Geometry: final body of the model. Coordinates: model frame, mm. A direction names the side the tool comes from. Round coordinates to 2 decimals unless told otherwise and drop trailing zeros. Loops run counter-clockwise (first coordinate to the right, second up) from the corner with the lowest first, then second, coordinate; pieces in that order, holes last. Notation, with made-up numbers: (16, 74) - (63, 74) arc R21 ccw to (63, 100) - close; hole circle Ø9 at (40.25, 81.25). An arc over 180 degrees is marked (long way). Answer as a JSON object with one key per item and string values. Group by question number.
Item 1: Section D-D (y = -3). Return the cut outline in (x, z).
Item 2: First-contact query: pin 1 (1 mm diameter, centred on x = -45, y = -4, fed in from +Z); pin 2 (1.5 mm diameter, centred on y = 30.5, z = 13, fed in from +X). Flat tips, straight axial feed; report the tip coordinate or a pass-through.
Item 3: Reachability of faces 4 (the face through (3.847, 40.286, 10.14)), 5 (the face through (-15, 38.5, 14)) from +Z, -Z, +X, -X, +Y, -Y: full face, straight path, thin tool, end or side. Return the list, or none.
Item 4: Section B-B (z = 10). Return the cut outline in (x, y).
Item 5: Line query: line 1 (Y direction, x = -22, z = 8.25); line 2 (Z direction, x = 2.5, y = -1); line 3 (X direction, y = 33.5, z = 13.5). Output: solid intervals per line, ascending.
Item 6: Section C-C (x = -7.5). Return the cut outline in (y, z).
Item 7: Section A-A (y = -41.75). Return the cut outline in (x, z).
Item 8: Draft query along X for faces 1 (the face through (-69.828, -1, 10)), 2 (the face through (3.847, -43.214, 10.14)), 3 (the face through (-25, -45, 10)). Return one class per face: released by +X, released by -X, zero draft, split by the parting line, or undercut.
```python
from build123d import *

# Parameters (mm, degrees)
F0_W      = 90
F0_H      = 90
F1_DEPTH  = 20
F2_W      = 70
F2_H      = 77
F3_DEPTH  = 12
F12_R     = 1.5
F13_DEPTH = 25


with BuildPart() as f1:
    # F0 (on Top) → F1 (new body)
    with BuildSketch(Plane.XY):
        with Locations((-24.827586, 0)):
            Rectangle(F0_W, F0_H)
    extrude(amount=F1_DEPTH)

    # F2 (on face) → F3 (cut)
    with BuildSketch(Plane.XY.offset(20)):
        with Locations((-14.827586, 0)):
            Rectangle(F2_W, F2_H)
    extrude(amount=-F3_DEPTH, mode=Mode.SUBTRACT)

    # F4 (on face) → F5 (revolve, cut)
    with BuildSketch(Plane(origin=(0, -38.5, 0), x_dir=(-1, 0, 0), z_dir=(0, 1, 0))):
        with BuildLine():
            Line((32.327586, 11.5), (32.327586, 15.5))
            ThreePointArc((32.327586, 15.5), (30.327586, 13.5), (32.327586, 11.5))
        make_face()
    revolve(axis=Axis((-32.327586, -38.5, 13.5), (0, 0, 1)), mode=Mode.SUBTRACT)

    # F6 (on face) → F7 (revolve, cut)
    with BuildSketch(Plane(origin=(0, -38.5, 0), x_dir=(-1, 0, 0), z_dir=(0, 1, 0))):
        with BuildLine():
            Line((-2.672414, 11.5), (-2.672414, 15.5))
            ThreePointArc((-2.672414, 15.5), (-4.672414, 13.5), (-2.672414, 11.5))
        make_face()
    revolve(axis=Axis((2.672414, -38.5, 13.5), (0, 0, 1)), mode=Mode.SUBTRACT)

    # F8 (on face) → F9 (revolve, cut)
    with BuildSketch(Plane.XZ.offset(-38.5)):
        with BuildLine():
            Line((2.672414, 15.5), (2.672414, 11.5))
            ThreePointArc((2.672414, 11.5), (4.672414, 13.5), (2.672414, 15.5))
        make_face()
    revolve(axis=Axis((2.672414, 38.5, 13.5), (0, 0, 1)), mode=Mode.SUBTRACT)

    # F10 (on face) → F11 (revolve, cut)
    with BuildSketch(Plane.XZ.offset(-38.5)):
        with BuildLine():
            Line((-32.327586, 11.5), (-32.327586, 15.5))
            ThreePointArc((-32.327586, 15.5), (-34.327586, 13.5), (-32.327586, 11.5))
        make_face()
    revolve(axis=Axis((-32.327586, 38.5, 13.5), (0, 0, 1)), mode=Mode.SUBTRACT)

    # F12 (on face) → F13 (cut)
    with BuildSketch(Plane.XY.offset(20)):
        with Locations((4.172414, -41.75)):
            Circle(F12_R)
        with Locations((4.172414, 41.75)):
            Circle(F12_R)
    extrude(amount=-F13_DEPTH, mode=Mode.SUBTRACT)


solid = f1.part
```
Values:
{
 "1": {"outline": "(-69.83, 0) - (20.17, 0) - (20.17, 8) - (-49.83, 8) - (-49.83, 20) - (-69.83, 20) - close"},
 "2": {"pin 1": "stops at z = 8", "pin 2": "stops at x = -49.83"},
 "3": {"face 4": "+Z, -Z", "face 5": "+Z, +X"},
 "4": {"outline": "(-69.83, -45) - (20.17, -45) - (20.17, -38.5) - (-49.83, -38.5) - (-49.83, 38.5) - (20.17, 38.5) - (20.17, 45) - (-69.83, 45) - close; hole circle Ø3 at (4.17, -41.75); hole circle Ø3 at (4.17, 41.75)"},
 "5": {"line 1": "y = -45 to -38.5, 38.5 to 45", "line 2": "z = 0 to 8", "line 3": "x = -69.83 to -49.83"},
 "6": {"outline": "(-45, 0) - (45, 0) - (45, 20) - (38.5, 20) - (38.5, 8) - (-38.5, 8) - (-38.5, 20) - (-45, 20) - close"},
 "7": {"outline": "(-69.83, 0) - (2.67, 0) - (2.67, 20) - (-69.83, 20) - close; (5.67, 0) - (20.17, 0) - (20.17, 20) - (5.67, 20) - close"},
 "8": {"face 1": "released by -X", "face 2": "undercut", "face 3": "zero draft"}
}
